Work out the finished part from the listing and answer in its coordinate system (mm). A direction names the side the tool comes from. Coordinates: 2 decimals unless noted, no trailing zeros. Order: outer loops, then holes, each group sorted by start corner. A loop starts at its lowest first (then second) coordinate and runs counter-clockwise, first axis right, second up. Notation, with made-up numbers: M 1,70.5 L 32,70.5 A19 cw 32,95.5 Z; hole C 26.25,-38 d5. An arc over 180 degrees is marked long. Use a Markdown table: item, result.
from build123d import *

# Parameters (mm, degrees)
BOSS_EXTRUDE1_DEPTH = 5
SKETCH3_R           = 5
BOSS_EXTRUDE2_DEPTH = 10
SKETCH4_R           = 2
CUT_EXTRUDE1_DEPTH  = 29
CHAMFER1_SIZE       = 0.5
CHAMFER2_SIZE       = 1


with BuildPart() as part:
    # Sketch1 → Revolve1 (revolve)
    with BuildSketch(Plane(origin=(0, 0, 0), x_dir=(1, 0, 0), z_dir=(0, 1, 0))):
        Polygon((0, 0), (0, 3), (-2, 3), (-2, 4), (-6, 4), (-6, 3), (-9, 3), (-9, 4), (-13, 4), (-13, 0), align=None)
    revolve(axis=Axis((8.879781421, 0, 0), (-1, 0, 0)))

    # Sketch2 → Boss-Extrude1 (add)
    with BuildSketch(Plane.ZY.offset(13)):
        Polygon((6.92820323, 0), (3.464101615, 6), (-3.464101615, 6), (-6.92820323, 0), (-3.464101615, -6), (3.464101615, -6), align=None)
    extrude(amount=BOSS_EXTRUDE1_DEPTH)

    # Sketch3 → Boss-Extrude2 (add)
    with BuildSketch(Plane.ZY.offset(18)):
        Circle(SKETCH3_R)
    extrude(amount=BOSS_EXTRUDE2_DEPTH)

    # Sketch4 → Cut-Extrude1 (cut, through all)
    with BuildSketch(Plane(origin=(0, 0, 0), x_dir=(0, 0, -1), z_dir=(1, 0, 0))):
        Circle(SKETCH4_R)
    extrude(amount=-CUT_EXTRUDE1_DEPTH, mode=Mode.SUBTRACT)

    # Chamfer1
    chamfer1_edges = [part.edges().sort_by_distance(p)[0] for p in [
        (-6, 0, 4),
        (-2, 0, 4),
        (0, 0, 3),
        (-28, 0, 2),
        (-9, 0, 4),
    ]]
    chamfer(chamfer1_edges, length=CHAMFER1_SIZE)

    # Chamfer2
    chamfer2_edges = [part.edges().sort_by_distance(p)[0] for p in [
        (-28, 0, -5),
    ]]
    chamfer(chamfer2_edges, length=CHAMFER2_SIZE)


solid = part.part
(1) A cutting plane is placed at C-C (x = -22). Determine the outline of the cut face in (y, z), then the cut area to 3 significant figures.
Conclusion:
| item | result |
|---|---|
| outline | C 0,0 d10; hole C 0,0 d4 |
| area | 66.0 mm2 |
(2) A cutting plane is placed at B-B (z = 6). Determine the outline of the cut face in (x, y), then the cut area to 3 significant figures.
Conclusion:
| item | result |
|---|---|
| outline | M -18,-1.61 L -13,-1.61 L -13,1.61 L -18,1.61 Z |
| area | 16.1 mm2 |
(3) Determine the mould class of faces 1 (the flat face through (-6, -1, -3)), 2 (the cylindrical face through (-22.44, -4.88, -1.08)), 3 (the flat face through (-13, 3, 3)), 4 (the cylindrical face through (-8, 0, 3)) for opening direction X: pulls with the +X half, pulls with the -X half, needs draft (parallel to the pull), parting line crosses it, or undercut.
Conclusion:
| item | result |
|---|---|
| face 1 | undercut |
| face 2 | needs draft |
| face 3 | pulls with the +X half |
| face 4 | undercut |
(4) Straight lines are drawn through the part: L1, parallel to X at y = 0.25, z = -3.25; L2, parallel to Y at x = -19, z = 0; L3, parallel to Y at x = -9.75, z = 0. For each, find the intervals that lie inside material, in ascending order.
Conclusion:
| item | result |
|---|---|
| L1 | -28 to -9, -6 to -2 |
| L2 | -5 to -2, 2 to 5 |
| L3 | -4 to -2, 2 to 4 |
(5) Which of the six approach directions +Z, -Z, +X, -X, +Y, -Y give full straight-line access (tool end or side, diameter ignored) to faces 5 (the cylindrical face through (-1, 0, 3)), 6 (the flat face through (-18, 5, 2)), 7 (the flat face through (-28, 2, 2))?
Conclusion:
| item | result |
|---|---|
| face 5 | +X |
| face 6 | -X |
| face 7 | +Z, -Z, -X, +Y, -Y |
(6) Given P1, Ø1, axis at x = -3, y = 3.5, coming from the +Z side; P2, Ø3, axis at x = -7, z = -2.5, coming from the +Y side; P3, Ø3, axis at x = -5.5, z = -2, coming from the -Y side; P4, Ø3.5, axis at y = 0, z = 0, coming from the +X side, each flat-ended and moving along its own axis, determine where each tip first touches the part or whether it passes through.
Conclusion:
| item | result |
|---|---|
| P1 | z = 2.65 |
| P2 | y = 3.38 |
| P3 | y = -3.97 |
| P4 | through |
(7) A cutting plane is placed at A-A (x = -10.75). Determine the outline of the cut face in (y, z), then the cut area to 3 significant figures.
Conclusion:
| item | result |
|---|---|
| outline | C 0,0 d8; hole C 0,0 d4 |
| area | 37.7 mm2 |
